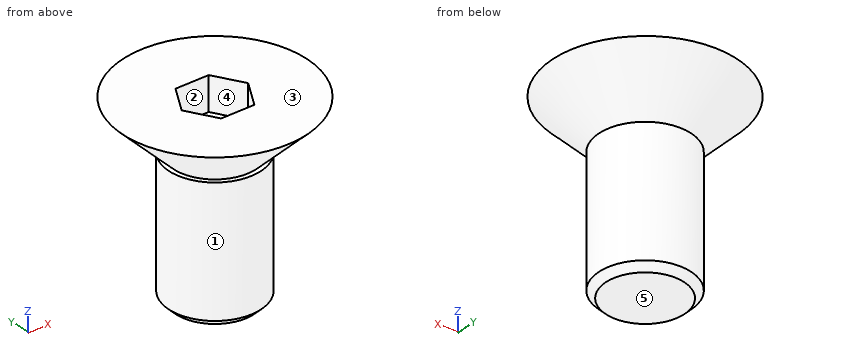
Solid Edge part; units mm, degrees
sketch "Sketch1" plane through (0, 0, 0) normal (0, 0, 1) x (1, 0, 0)
  circle A0 centre (0, 0) radius 8
extrude "Protrusion1" add sketch "Sketch1" along normal blind 4.4
sketch "Sketch2" plane through (0, 0, 0) normal (0, 0, -1) x (1, 0, 0)
  circle A0 centre (0, 0) radius 4
extrude "Protrusion2" add sketch "Sketch2" along normal blind 11.6
sketch "Sketch3" plane through (0, 0, -11.6) normal (0, 0, -1) x (1, 0, 0)
  circle A0 centre (0, 0) radius 3.9997
extrude "Cutout1" cut sketch "Sketch3" against normal blind 11.5884 flip side to cut
chamfer "Chamfer_1" distance 0.6 angle 45 1 edges at (-3.9997, 0, -11.6)
sketch "Sketch4" plane through (0, 0, 4.4) normal (0, 0, 1) x (1, 0, 0)
  line L0 (-1.4434, 2.5) -> (1.4434, 2.5)
  line L1 (2.8868, 0) -> (1.4434, 2.5)
  line L2 (1.4434, -2.5) -> (2.8868, 0)
  line L3 (-1.4434, -2.5) -> (1.4434, -2.5)
  line L4 (-2.8868, 0) -> (-1.4434, -2.5)
  line L5 (-1.4434, 2.5) -> (-2.8868, 0)
extrude "Cutout2" cut sketch "Sketch4" against normal blind 2.9333
sketch "Sketch5" plane through (0, 0, 0) normal (0, -1, 0) x (1, 0, 0)
  line L0 (8, 4.4) -> (3.6, 0)
  line L1 (3.6, 0) -> (8, 0)
  line L2 (8, 0) -> (8, 4.4)
revolve "RevolvedCutout1" cut sketch "Sketch5" angle 360 about axis through (0, 0, 14.0017) along (0, 0, -1)
properties part number "24101875"
The listing builds one solid part. Answer for the finished solid, in the listing's coordinates (mm). Face numbers are marked on the shaded views. A direction names the side the tool comes from. Coordinates: 2 decimals unless noted, no trailing zeros. Order: outer loops, then holes, each group sorted by start corner. A loop starts at its lowest first (then second) coordinate and runs counter-clockwise, first axis right, second up. Notation, with made-up numbers: (75.25, 15.5) -> (122.25, 15.5) arc R25 cw to (122.25, 51.5) -> close; hole circle Ø3 at (-23, 85). An arc over 180 degrees is marked (long way). Answer in a Markdown table with one row per item. Add a question column.
Item 1: Which of the six approach directions +Z, -Z, +X, -X, +Y, -Y give full straight-line access (tool end or side, diameter ignored) to the marked faces 4 and 5?
Item 2: Each of these flat-tipped pins is pushed along its axis until it touches: P1, Ø2.5, axis at x = -0.5, z = 3, coming from the -Y side; P2, Ø1, axis at x = 5, y = -1.5, coming from the -Z side; P3, Ø4, axis at x = -2.5, z = -1.5, coming from the -Y side. Where does it stop, or does it pass through?
Item 3: Find section C-C (z = -5). Write down the section's boundary in (x, y).
Item 4: Find the intervals of material crossed by L1, parallel to X at y = -1.75, z = 2.5; L2, parallel to Z at x = -6.25, y = -1.75; L3, parallel to Y at x = -0.25, z = 2, in increasing order. Write a range as from..to.
Item 5: Find section B-B (z = 0.75). Write down the section's boundary in (x, y).
Item 6: Determine the mould class of the marked faces 1, 2 and 3 for opening direction X: +X half, -X half, draft (parallel to the pull), parting line (faces both ways), or undercut.
Result set:
| question | item | result |
|---|---|---|
| 1 | face 4 | +Z |
| 1 | face 5 | -Z, +X, -X, +Y, -Y |
| 2 | P1 | stops at y = -7.84 |
| 2 | P2 | stops at z = 1.12 |
| 2 | P3 | stops at y = -3.97 |
| 3 | outline | circle Ø8 at (0, 0) |
| 4 | L1 | x = -5.84..-1.88, 1.88..5.84 |
| 4 | L2 | z = 2.89..4.4 |
| 4 | L3 | y = -5.59..-2.5, 2.5..5.59 |
| 5 | outline | circle Ø8.7 at (0, 0) |
| 6 | face 1 | parting line |
| 6 | face 2 | undercut |
| 6 | face 3 | draft |
